```python
from build123d import *

# Parameters (mm, degrees)
F1_DEPTH = 10.16


with BuildPart() as f1:
    # F0 (on Top) → F1 (new body)
    with BuildSketch(Plane.XY):
        Polygon((19.05, 0), (0, 0), (0, -19.05), (10.16, -19.05), (10.16, -31.75), (0, -31.75), (0, -44.45), (10.16, -44.45), (10.16, -57.15), (0, -57.15), (0, -69.85), (10.16, -69.85), (10.16, -82.55), (0, -82.55), (0, -101.6), (19.05, -101.6), (19.05, -91.44), (31.75, -91.44), (31.75, -101.6), (44.45, -101.6), (44.45, -91.44), (57.15, -91.44), (57.15, -101.6), (69.85, -101.6), (69.85, -91.44), (82.55, -91.44), (82.55, -101.6), (95.25, -101.6), (95.25, -91.44), (107.95, -91.44), (107.95, -101.6), (120.65, -101.6), (120.65, -91.44), (133.35, -91.44), (133.35, -101.6), (146.05, -101.6), (146.05, -91.44), (158.75, -91.44), (158.75, -101.6), (171.45, -101.6), (171.45, -91.44), (184.15, -91.44), (184.15, -101.6), (203.2, -101.6), (203.2, -82.55), (193.04, -82.55), (193.04, -69.85), (203.2, -69.85), (203.2, -57.15), (193.04, -57.15), (193.04, -44.45), (203.2, -44.45), (203.2, -31.75), (193.04, -31.75), (193.04, -19.05), (203.2, -19.05), (203.2, 0), (184.15, 0), (184.15, -10.16), (171.45, -10.16), (171.45, 0), (158.75, 0), (158.75, -10.16), (146.05, -10.16), (146.05, 0), (133.35, 0), (133.35, -10.16), (120.65, -10.16), (120.65, 0), (107.95, 0), (107.95, -10.16), (95.25, -10.16), (95.25, 0), (82.55, 0), (82.55, -10.16), (69.85, -10.16), (69.85, 0), (57.15, 0), (57.15, -10.16), (44.45, -10.16), (44.45, 0), (31.75, 0), (31.75, -10.16), (19.05, -10.16), align=None)
        with BuildLine():
            ThreePointArc((63.5, -20.32), (64.615923, -17.625923), (67.31, -16.51))
            Line((67.31, -16.51), (135.89, -16.51))
            ThreePointArc((135.89, -16.51), (138.584077, -17.625923), (139.7, -20.32))
            Line((139.7, -20.32), (139.7, -22.86))
            ThreePointArc((139.7, -22.86), (138.584077, -25.554077), (135.89, -26.67))
            Line((135.89, -26.67), (67.31, -26.67))
            ThreePointArc((67.31, -26.67), (64.615923, -25.554077), (63.5, -22.86))
            Line((63.5, -22.86), (63.5, -20.32))
        make_face(mode=Mode.SUBTRACT)
    extrude(amount=F1_DEPTH)


solid = f1.part
```
Work out the finished part from the listing and answer in its coordinate system (mm). A direction names the side the tool comes from. Coordinates: 2 decimals unless noted, no trailing zeros. Loops run counter-clockwise (first coordinate to the right, second up) from the corner with the lowest first, then second, coordinate; pieces in that order, holes last. Notation, with made-up numbers: M -26,-34 L 15,-34 A15 ccw 15,-24 Z; hole C 21.25,77.5 d5. An arc over 180 degrees is marked long. Use CSV: the item, a comma, the result in double quotes. Start each with the question number.
(1) Given pin 1 Ø12 at (x, y) = (53, -62.5) entering from -Z; pin 2 Ø5 at (y, z) = (-23.5, 4) entering from +X; pin 3 Ø5 at (y, z) = (-28, 7) entering from -X; pin 4 Ø5 at (x, z) = (181, 3.5) entering from -Y, each flat-ended and moving along its own axis, determine where each tip first touches the part or whether it passes through.
(2) Consider line 1 (Y direction, x = 194, z = 7.25); line 2 (Y direction, x = 92.5, z = 6.25); line 3 (Y direction, x = 100, z = 0.75). Determine where each line is inside the solid, lowest interval first.
(3) For faces 4 (the face through (198, -31.75, 5)), 5 (the face through (140, -101.6, 5)), 6 (the face through (178, -91.44, 5)), 7 (the face through (19.05, -5, 5)), 8 (the face through (10.16, -25, 5)), determine the directions among +Z, -Z, +X, -X, +Y, -Y from which every point of the face is accessible in a straight line to the end or side of a thin tool.
(4) Find section A-A, the plane x = 123. Give the vertices of the cut face in (y, z), then the cut area to 3 significant figures.
(5) Find section C-C, the plane y = -51. Give the vertices of the cut face in (x, z), then the cut area to 3 significant figures.
(6) Find section B-B, the plane x = 22. Give the vertices of the cut face in (y, z), then the cut area to 3 significant figures.
(7) For a pull along Y with two mould halves and no side action, classify faces 1 (the face through (178, -10.16, 5)), 2 (the face through (184.15, -96, 5)), 3 (the face through (138.554, -17.596, 5.009)) as +Y half, -Y half, draft (parallel to the pull), parting line (faces both ways), or undercut.
Recorded:
1,pin 1,"stops at z = 0"
1,pin 2,"stops at x = 193.04"
1,pin 3,"stops at x = 10.16"
1,pin 4,"stops at y = -91.44"
2,line 1,"y = -101.6 to -82.55, -69.85 to -57.15, -44.45 to -31.75, -19.05 to 0"
2,line 2,"y = -101.6 to -26.67, -16.51 to 0"
2,line 3,"y = -91.44 to -26.67, -16.51 to -10.16"
3,face 4,"+Z, -Z, +X"
3,face 5,"+Z, -Z, +X, -X, -Y"
3,face 6,"+Z, -Z, -Y"
3,face 7,"+Z, -Z, +Y"
3,face 8,"+Z, -Z, -X"
4,outline,"M -91.44,0 L -26.67,0 L -26.67,10.16 L -91.44,10.16 Z; M -16.51,0 L -10.16,0 L -10.16,10.16 L -16.51,10.16 Z"
4,area,"723 mm^2"
5,outline,"M 10.16,0 L 193.04,0 L 193.04,10.16 L 10.16,10.16 Z"
5,area,"1,860 mm^2"
6,outline,"M -91.44,0 L -10.16,0 L -10.16,10.16 L -91.44,10.16 Z"
6,area,"826 mm^2"
7,face 1,"+Y half"
7,face 2,"draft"
7,face 3,"undercut"
